Autodesk Inventor part; units mm, degrees
ref_plane "YZ Plane" through (0, 0, 0) normal (1, 0, 0) x (0, 1, 0)
ref_plane "XZ Plane" through (0, 0, 0) normal (0, 1, 0) x (-1, 0, 0)
ref_plane "XY Plane" through (0, 0, 0) normal (0, 0, 1) x (1, 0, 0)
sketch "Szkic1" plane through (0, 0, 0) normal (0, 0, 1) x (1, 0, 0)
  line L0 (0, 2) -> (0, 40)
  line L1 (0, 40) -> (2, 40)
  line L2 (2, 40) -> (2, 4)
  line L3 (4, 2) -> (40, 2)
  line L4 (40, 2) -> (40, 0)
  line L5 (40, 0) -> (2, 0)
  arc A0 (0, 2) -> (2, 0) centre (2, 2) ccw
  arc A1 (2, 4) -> (4, 2) centre (4, 4) ccw
  point P0 (0, 0)
  point P1 (2, 2)
  dimension "d0" = 40
  dimension "d1" = 2
  dimension "d2" = 38
  dimension "d3" = 38
  dimension "d4" = 2
extrude "Wyciągnięcie proste1" add sketch "Szkic1" along normal blind 40
sketch "Szkic2" plane through (2, 4, 0) normal (1, 0, 0) x (0, 0, -1)
  line L0 (0, 0) -> (-40, 0)
  line L1 (-20, 0) -> (-20, 36)
  line L2 (0, 36) -> (-40, 36)
  line L3 (-20, 18) -> (-40, 18)
  line L4 (-40, 0) -> (-40, 36)
  line L5 (-20, 18) -> (0, 18)
  line L6 (-40, 18) -> (-40, 27)
  line L7 (-40, 27) -> (-30, 27)
  line L8 (0, 0) -> (0, 36)
  line L9 (0, 27) -> (-10, 27)
  line L10 (-20, 18) -> (-20, 9)
  point P0 (0, -4)
  dimension "d13" = 9
  dimension "d14" = 30
  dimension "d16" = 9
  dimension "d17" = 20
  dimension "d18" = 9
sketch "Szkic3" plane through (4, 2, 0) normal (0, 1, 0) x (1, 0, 0)
  line L0 (0, 0) -> (0, -40)
  line L1 (0, -40) -> (0, -20)
  line L2 (0, -20) -> (9, -20)
  line L3 (36, -40) -> (0, -40)
  line L4 (18, -40) -> (18, 0)
  line L5 (36, 0) -> (0, 0)
  line L6 (18, -20) -> (36, -20)
  line L7 (36, 0) -> (36, -40)
  line L8 (27, -20) -> (27, -30)
  line L9 (27, -20) -> (27, -10)
  point P0 (-4, 0)
  dimension "d19" = 9
  dimension "d20" = 10
  dimension "d21" = 10
hole "Otwór1" at (2, 31, 30) at (2, 31, 10) at (2, 13, 20) direction (-1, 0, 0) diameter 8 end through all countersink diameter 10 countersink angle 90
hole "Otwór2" at (13, 2, 20) at (31, 2, 30) at (31, 2, 10) direction (0, -1, 0) diameter 8 end through all countersink diameter 10 countersink angle 90
properties part number "katownik_lacznikowy_40_40_40"
Can you work these out from the model? Positions are in its coordinate system, mm. A direction names the side the tool comes from. Coordinates: 2 decimals unless noted, no trailing zeros. Order: outer loops, then holes, each group sorted by start corner. A loop starts at its lowest first (then second) coordinate and runs counter-clockwise, first axis right, second up.
1. If we section it at D-D (y = 31): Please give me the cut outline in (x, z).
2. For faces 1 (the face through (15.4, 0.5, 16.8)), 2 (the face through (22, 2, 20)), which set-ups out of +Z, -Z, +X, -X, +Y, -Y let a thin tool reach every point of the face, with its end or its side?
3. Thinking about a two-plate mould opening in X: for faces 3 (the face through (2.6, 2.57, 19.72)), 4 (the face through (1, 11, 0)), 5 (the face through (27.034, 0.493, 29.479)), 6 (the face through (27.034, 0.493, 9.479)), which applies, +X half, -X half, draft (parallel to the pull), parting line (faces both ways), or undercut?
4. If we section it at A-A (y = 13): Please give me the cut outline in (x, z).
5. I need wall thicknesses on line 1 (Z direction, x = 31, y = 0.65); line 2 (Z direction, x = 13, y = 0.3); line 3 (Y direction, x = 38, z = 24). Which ranges of each line are inside material? Lowest first, please.
6. I'm going to push flat-ended pins straight in: pin 1 (9 mm diameter, centred on y = 31, z = 10, fed in from +X); pin 2 (3 mm diameter, centred on x = 11.5, z = 34.5, fed in from +Y); pin 3 (10.5 mm diameter, centred on y = 13, z = 20, fed in from +X). Where does each tip first touch, or does it pass through?
7. If we section it at B-B (z = 20): Please give me the cut outline in (x, y).
Entries:
1. outline: (0, 0) - (2, 0) - (2, 5) - (1, 6) - (0, 6) - close; (0, 14) - (1, 14) - (2, 15) - (2, 25) - (1, 26) - (0, 26) - close; (0, 34) - (1, 34) - (2, 35) - (2, 40) - (0, 40) - close
2. face 1: +Y, -Y
2. face 2: +Z, -Z, +X, +Y
3. face 3: +X half
3. face 4: draft
3. face 5: undercut
3. face 6: undercut
4. outline: (0, 0) - (2, 0) - (2, 15) - (1, 16) - (0, 16) - close; (0, 24) - (1, 24) - (2, 25) - (2, 40) - (0, 40) - close
5. line 1: z = 0 to 6, 14 to 26, 34 to 40
5. line 2: z = 0 to 16, 24 to 40
5. line 3: y = 0 to 2
6. pin 1: stops at x = 1.5
6. pin 2: stops at y = 2
6. pin 3: stops at x = 2
7. outline: (0, 2) arc R2 ccw to (2, 0) - (9, 0) - (9, 1) - (8, 2) - (4, 2) arc R2 cw to (2, 4) - (2, 8) - (1, 9) - (0, 9) - close; (0, 17) - (1, 17) - (2, 18) - (2, 40) - (0, 40) - close; (17, 0) - (40, 0) - (40, 2) - (18, 2) - (17, 1) - close
